The model under review builds one solid part; all positions refer to its coordinate system, in mm. Face numbers are marked on the shaded views. A direction names the side the tool comes from. Coordinates: 2 decimals unless noted, no trailing zeros. Order: outer loops, then holes, each group sorted by start corner. A loop starts at its lowest first (then second) coordinate and runs counter-clockwise, first axis right, second up.
```python
from build123d import *

# Parameters (mm, degrees)
RESSALTO_EXTRUS_O1_DEPTH = 2.5
ESBO_O2_R                = 0.5
CORTE_EXTRUS_O1_DEPTH    = 27.968129338
CORTE_EXTRUS_O2_DEPTH    = 4


with BuildPart() as part:
    # Esboço1 → Ressalto-extrusão1 (new, symmetric)
    with BuildSketch(Plane(origin=(0, 0, 0), x_dir=(1, 0, 0), z_dir=(0, 1, 0))):
        with BuildLine():
            Line((-25.2, 0), (-19.2, 0))
            ThreePointArc((-19.2, 0), (-16, -3.2), (-12.8, 0))
            Line((-12.8, 0), (-11.2, 0))
            ThreePointArc((-11.2, 0), (-8, -3.2), (-4.8, 0))
            Line((-4.8, 0), (-3.2, 0))
            ThreePointArc((-3.2, 0), (0, -3.2), (3.2, 0))
            Line((3.2, 0), (4.8, 0))
            ThreePointArc((4.8, 0), (8, -3.2), (11.2, 0))
            Line((11.2, 0), (12.8, 0))
            ThreePointArc((12.8, 0), (16, -3.2), (19.2, 0))
            Line((19.2, 0), (25.2, 0))
            Line((25.2, 0), (25.2, -8.2))
            Line((25.2, -8.2), (-25.2, -8.2))
            Line((-25.2, -8.2), (-25.2, 0))
        make_face()
    extrude(amount=RESSALTO_EXTRUS_O1_DEPTH, both=True)

    # Esboço2 → Corte-extrusão1 (cut, through all)
    with BuildSketch(Plane(origin=(0, 2.5, 0), x_dir=(1, 0, 0), z_dir=(0, 1, 0))):
        with Locations((-12, 0)):
            Circle(ESBO_O2_R)
        with Locations((-4, 0)):
            Circle(ESBO_O2_R)
        with Locations((4, 0)):
            Circle(ESBO_O2_R)
        with Locations((12, 0)):
            Circle(ESBO_O2_R)
    extrude(amount=-CORTE_EXTRUS_O1_DEPTH, mode=Mode.SUBTRACT)

    # Esboço3 → Corte-extrusão2 (cut)
    with BuildSketch(Plane(origin=(0, 2.5, 0), x_dir=(1, 0, 0), z_dir=(0, 1, 0))):
        with BuildLine():
            Line((-23.7, 0), (-20.7, 0))
            Line((-20.7, 0), (-20.7, -4))
            ThreePointArc((-20.7, -4), (-19.2, -5.5), (-20.7, -7))
            Line((-20.7, -7), (-21.7, -7))
            ThreePointArc((-21.7, -7), (-23.114213562, -6.414213562), (-23.7, -5))
            Line((-23.7, -5), (-23.7, 0))
        make_face()
        with BuildLine():
            Line((20.7, 0), (20.7, -4))
            ThreePointArc((20.7, -4), (19.2, -5.5), (20.7, -7))
            Line((20.7, -7), (21.7, -7))
            ThreePointArc((21.7, -7), (23.114213562, -6.414213562), (23.7, -5))
            Line((23.7, -5), (23.7, 0))
            Line((23.7, 0), (20.7, 0))
        make_face()
    extrude(amount=-CORTE_EXTRUS_O2_DEPTH, mode=Mode.SUBTRACT)


solid = part.part
```
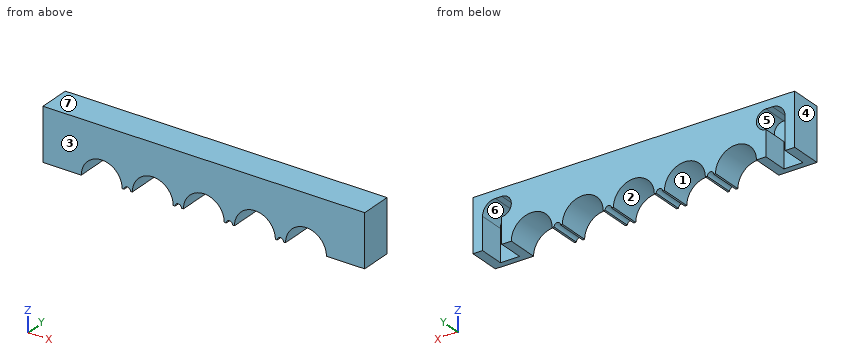
(1) We need section D-D, the plane z = 5.5. Write out the cut boundary in (x, y).
A:
outline: (-25.2, -2.5) - (25.2, -2.5) - (25.2, 2.5) - (23.64, 2.5) - (23.64, -1.5) - (19.2, -1.5) - (19.2, 2.5) - (-19.2, 2.5) - (-19.2, -1.5) - (-23.64, -1.5) - (-23.64, 2.5) - (-25.2, 2.5) - close
(2) We need section B-B, the plane y = -2. Write out the cut boundary in (x, z).
A:
outline: (-25.2, 0) - (-19.2, 0) arc R3.2 cw to (-12.8, 0) - (-12.5, 0) arc R0.5 cw to (-11.5, 0) - (-11.2, 0) arc R3.2 cw to (-4.8, 0) - (-4.5, 0) arc R0.5 cw to (-3.5, 0) - (-3.2, 0) arc R3.2 cw to (3.2, 0) - (3.5, 0) arc R0.5 cw to (4.5, 0) - (4.8, 0) arc R3.2 cw to (11.2, 0) - (11.5, 0) arc R0.5 cw to (12.5, 0) - (12.8, 0) arc R3.2 cw to (19.2, 0) - (25.2, 0) - (25.2, 8.2) - (-25.2, 8.2) - close
(3) We need section C-C, the plane x = -4. Write out the cut boundary in (y, z).
A:
outline: (-2.5, 0.5) - (2.5, 0.5) - (2.5, 8.2) - (-2.5, 8.2) - close
(4) For pin 1 Ø0.8 at (x, y) = (21, 1.5) entering from -Z; pin 2 Ø3 at (x, z) = (8.5, 1) entering from +Y; pin 3 Ø1.1 at (x, y) = (-21.5, 1) entering from -Z; pin 4 Ø1.3 at (x, z) = (-22.5, 2.5) entering from +Y, all flat-tipped, find the tip position at first contact; note any pin that passes through.
A:
pin 1: stops at z = 0
pin 2: passes through
pin 3: stops at z = 6.97
pin 4: stops at y = -1.5
(5) Machinability: for the marked faces 5, 6 and 7, which of the approach directions +Z, -Z, +X, -X, +Y, -Y give a long, thin tool a straight path to every point of the face, cutting with its end or side? Answer none if there is none.
A:
face 5: +Y
face 6: -Z, +Y
face 7: +Z, +X, -X, +Y, -Y
(6) We need section A-A, the plane z = 1.5. Count the separate pieces of the cut face and the enclosed holes in it, and give its area (3 significant figures).
A:
separate pieces: 6
enclosed holes: 0
area: 86.7 mm2
(7) Draft analysis for pull direction X (two halves, no side actions). For the marked faces 1, 2, 3 and 4, state which applies: released by +X, released by -X, zero draft, split by the parting line, or undercut.
A:
face 1: undercut
face 2: undercut
face 3: zero draft
face 4: released by -X
(8) Wall thickness on probe 1 along X at (y, z) = (-0.2, 5); probe 2 along X at (y, z) = (-1.65, 1.5); probe 3 along Z at (x, y) = (4, 1.55): over which ranges is each line inside the solid? List them lowest first.
A:
probe 1: x = -25.2 to -23.7, -19.29 to 19.29, 23.7 to 25.2
probe 2: x = -25.2 to -18.83, -13.17 to -10.83, -5.17 to -2.83, 2.83 to 5.17, 10.83 to 13.17, 18.83 to 25.2
probe 3: z = 0.5 to 8.2
